from build123d import *

# Parameters (mm, degrees)
P_IDAT_VYSUNUT_M1_DEPTH      = 42
SKICA7_W                     = 10
SKICA7_H                     = 6
P_IDAT_VYSUNUT_M2_DEPTH      = 10
SKICA8_R                     = 3
ODEBRAT_VYSUNUT_M4_DEPTH     = 3
SKICA9_R                     = 1.55
ODEBRAT_VYSUNUT_M5_DEPTH     = 3
LINPOLE1_COUNT               = 2
LINPOLE1_PITCH               = 43
KRUHOV_POLE1_COUNT           = 4
KRUHOV_POLE1_COPY_1_SKETCH_W = 10
KRUHOV_POLE1_COPY_1_SKETCH_H = 6
KRUHOV_POLE1_COPY_1_DEPTH    = 10
KRUHOV_POLE1_COPY_2_SKETCH_W = 10
KRUHOV_POLE1_COPY_2_SKETCH_H = 6
KRUHOV_POLE1_COPY_2_DEPTH    = 10
KRUHOV_POLE1_COPY_3_SKETCH_W = 10
KRUHOV_POLE1_COPY_3_SKETCH_H = 6
KRUHOV_POLE1_COPY_3_DEPTH    = 10
KRUHOV_POLE1_COPY_4_SKETCH_R = 3
KRUHOV_POLE1_COPY_4_DEPTH    = 3
KRUHOV_POLE1_COPY_5_SKETCH_R = 3
KRUHOV_POLE1_COPY_5_DEPTH    = 3
KRUHOV_POLE1_COPY_6_SKETCH_R = 3
KRUHOV_POLE1_COPY_6_DEPTH    = 3
KRUHOV_POLE1_COPY_7_SKETCH_R = 1.55
KRUHOV_POLE1_COPY_7_DEPTH    = 3
KRUHOV_POLE1_COPY_8_SKETCH_R = 1.55
KRUHOV_POLE1_COPY_8_DEPTH    = 3
KRUHOV_POLE1_COPY_9_SKETCH_R = 1.55
KRUHOV_POLE1_COPY_9_DEPTH    = 3
ZAOBLIT3_R                   = 2


with BuildPart() as part:
    # Skica2 → Přidat vysunutím1 (new body)
    with BuildSketch(Plane.XY):
        with BuildLine():
            Line((3, 0), (110, 0))
            ThreePointArc((110, 0), (112.121320344, -0.878679656), (113, -3))
            Line((113, -3), (113, -110))
            ThreePointArc((113, -110), (112.121320344, -112.121320344), (110, -113))
            Line((110, -113), (3, -113))
            ThreePointArc((3, -113), (0.878679656, -112.121320344), (0, -110))
            Line((0, -110), (0, -3))
            ThreePointArc((0, -3), (0.878679656, -0.878679656), (3, 0))
        make_face()
        with BuildLine():
            Line((1, -3), (1, -110))
            ThreePointArc((1, -110), (1.585786438, -111.414213562), (3, -112))
            Line((3, -112), (110, -112))
            ThreePointArc((110, -112), (111.414213562, -111.414213562), (112, -110))
            Line((112, -110), (112, -3))
            ThreePointArc((112, -3), (111.414213562, -1.585786438), (110, -1))
            Line((110, -1), (3, -1))
            ThreePointArc((3, -1), (1.585786438, -1.585786438), (1, -3))
        make_face(mode=Mode.SUBTRACT)
    extrude(amount=P_IDAT_VYSUNUT_M1_DEPTH)

    # Skica7 → Přidat vysunutím2 (add)
    with BuildSketch(Plane(origin=(0, 0, 0), x_dir=(1, 0, 0), z_dir=(0, 1, 0))):
        with Locations((35, -3)):
            Rectangle(SKICA7_W, SKICA7_H)
    p_idat_vysunut_m2 = extrude(amount=P_IDAT_VYSUNUT_M2_DEPTH)

    # Skica8 → Odebrat vysunutím4 (cut)
    with BuildSketch(Plane.XY.offset(6)):
        with Locations((35, 5)):
            Circle(SKICA8_R)
    odebrat_vysunut_m4 = extrude(amount=-ODEBRAT_VYSUNUT_M4_DEPTH, mode=Mode.SUBTRACT)

    # Skica9 → Odebrat vysunutím5 (cut)
    with BuildSketch(Plane.XY.offset(3)):
        with Locations((35, 5)):
            Circle(SKICA9_R)
    odebrat_vysunut_m5 = extrude(amount=-ODEBRAT_VYSUNUT_M5_DEPTH, mode=Mode.SUBTRACT)

    # LinPole1: Přidat vysunutím2, Odebrat vysunutím4, Odebrat vysunutím5 ×2
    with Locations(*[(i * LINPOLE1_PITCH, 0, 0) for i in range(1, LINPOLE1_COUNT)]):
        add(p_idat_vysunut_m2)
        add(odebrat_vysunut_m4, mode=Mode.SUBTRACT)
        add(odebrat_vysunut_m5, mode=Mode.SUBTRACT)

    # Kruhové pole1: Přidat vysunutím2, Odebrat vysunutím4, Odebrat vysunutím5 ×4 about axis
    kruhov_pole1_axis = Axis((56.5, -56.5, 0), (0, 0, 1))
    for i in range(1, KRUHOV_POLE1_COUNT):
        add(p_idat_vysunut_m2.rotate(kruhov_pole1_axis, i * 360 / KRUHOV_POLE1_COUNT))
        add(odebrat_vysunut_m4.rotate(kruhov_pole1_axis, i * 360 / KRUHOV_POLE1_COUNT), mode=Mode.SUBTRACT)
        add(odebrat_vysunut_m5.rotate(kruhov_pole1_axis, i * 360 / KRUHOV_POLE1_COUNT), mode=Mode.SUBTRACT)

    # Kruhové pole1 copy 1 sketch → Kruhové pole1 copy 1 (add)
    with BuildSketch(Plane(origin=(0, -70, 0), x_dir=(0, 1, 0), z_dir=(-1, 0, 0))):
        with Locations((35, -3)):
            Rectangle(KRUHOV_POLE1_COPY_1_SKETCH_W, KRUHOV_POLE1_COPY_1_SKETCH_H)
    extrude(amount=KRUHOV_POLE1_COPY_1_DEPTH)

    # Kruhové pole1 copy 2 sketch → Kruhové pole1 copy 2 (add)
    with BuildSketch(Plane(origin=(70, -113, 0), x_dir=(-1, 0, 0), z_dir=(0, -1, 0))):
        with Locations((35, -3)):
            Rectangle(KRUHOV_POLE1_COPY_2_SKETCH_W, KRUHOV_POLE1_COPY_2_SKETCH_H)
    extrude(amount=KRUHOV_POLE1_COPY_2_DEPTH)

    # Kruhové pole1 copy 3 sketch → Kruhové pole1 copy 3 (add)
    with BuildSketch(Plane(origin=(113, -43, 0), x_dir=(0, -1, 0), z_dir=(1, 0, 0))):
        with Locations((35, -3)):
            Rectangle(KRUHOV_POLE1_COPY_3_SKETCH_W, KRUHOV_POLE1_COPY_3_SKETCH_H)
    extrude(amount=KRUHOV_POLE1_COPY_3_DEPTH)

    # Kruhové pole1 copy 4 sketch → Kruhové pole1 copy 4 (cut)
    with BuildSketch(Plane(origin=(0, -70, 6), x_dir=(0, 1, 0), z_dir=(0, 0, 1))):
        with Locations((35, 5)):
            Circle(KRUHOV_POLE1_COPY_4_SKETCH_R)
    extrude(amount=-KRUHOV_POLE1_COPY_4_DEPTH, mode=Mode.SUBTRACT)

    # Kruhové pole1 copy 5 sketch → Kruhové pole1 copy 5 (cut)
    with BuildSketch(Plane(origin=(70, -113, 6), x_dir=(-1, 0, 0), z_dir=(0, 0, 1))):
        with Locations((35, 5)):
            Circle(KRUHOV_POLE1_COPY_5_SKETCH_R)
    extrude(amount=-KRUHOV_POLE1_COPY_5_DEPTH, mode=Mode.SUBTRACT)

    # Kruhové pole1 copy 6 sketch → Kruhové pole1 copy 6 (cut)
    with BuildSketch(Plane(origin=(113, -43, 6), x_dir=(0, -1, 0), z_dir=(0, 0, 1))):
        with Locations((35, 5)):
            Circle(KRUHOV_POLE1_COPY_6_SKETCH_R)
    extrude(amount=-KRUHOV_POLE1_COPY_6_DEPTH, mode=Mode.SUBTRACT)

    # Kruhové pole1 copy 7 sketch → Kruhové pole1 copy 7 (cut)
    with BuildSketch(Plane(origin=(0, -70, 3), x_dir=(0, 1, 0), z_dir=(0, 0, 1))):
        with Locations((35, 5)):
            Circle(KRUHOV_POLE1_COPY_7_SKETCH_R)
    extrude(amount=-KRUHOV_POLE1_COPY_7_DEPTH, mode=Mode.SUBTRACT)

    # Kruhové pole1 copy 8 sketch → Kruhové pole1 copy 8 (cut)
    with BuildSketch(Plane(origin=(70, -113, 3), x_dir=(-1, 0, 0), z_dir=(0, 0, 1))):
        with Locations((35, 5)):
            Circle(KRUHOV_POLE1_COPY_8_SKETCH_R)
    extrude(amount=-KRUHOV_POLE1_COPY_8_DEPTH, mode=Mode.SUBTRACT)

    # Kruhové pole1 copy 9 sketch → Kruhové pole1 copy 9 (cut)
    with BuildSketch(Plane(origin=(113, -43, 3), x_dir=(0, -1, 0), z_dir=(0, 0, 1))):
        with Locations((35, 5)):
            Circle(KRUHOV_POLE1_COPY_9_SKETCH_R)
    extrude(amount=-KRUHOV_POLE1_COPY_9_DEPTH, mode=Mode.SUBTRACT)

    # Zaoblit3
    zaoblit3_edges = [part.edges().sort_by_distance(p)[0] for p in [
        (83, -113, 3),
        (73, -113, 3),
        (83, -123, 3),
        (73, -123, 3),
        (0, -83, 3),
        (0, -73, 3),
        (-10, -83, 3),
        (-10, -73, 3),
        (113, -73, 3),
        (113, -83, 3),
        (123, -73, 3),
        (123, -83, 3),
        (40, -113, 3),
        (30, -113, 3),
        (40, -123, 3),
        (30, -123, 3),
        (0, -40, 3),
        (0, -30, 3),
        (-10, -40, 3),
        (-10, -30, 3),
        (30, 0, 3),
        (40, 0, 3),
        (30, 10, 3),
        (40, 10, 3),
        (73, 0, 3),
        (83, 0, 3),
        (73, 10, 3),
        (83, 10, 3),
        (113, -30, 3),
        (113, -40, 3),
        (123, -30, 3),
        (123, -40, 3),
    ]]
    fillet(zaoblit3_edges, radius=ZAOBLIT3_R)


solid = part.part
Verification items for the finished model (mm, model axes). A direction names the side the tool comes from. Coordinates: 2 decimals unless noted, no trailing zeros. Order: outer loops, then holes, each group sorted by start corner. A loop starts at its lowest first (then second) coordinate and runs counter-clockwise, first axis right, second up.
1. Scan lines: line 1 (X direction, y = -78, z = 4.1); line 2 (Y direction, x = -5, z = 1.7); line 3 (X direction, y = -35, z = 0.9). Record each from-to range of solid material in increasing order.
Results found:
line 1: x = -10 to -8, -2 to 1, 112 to 115, 121 to 123
line 2: y = -83 to -79.55, -76.45 to -73, -40 to -36.55, -33.45 to -30
line 3: x = -10 to -6.55, -3.45 to 1, 112 to 116.45, 119.55 to 123
2. Sectioned sample at A-A, the plane x = 6.5. Record the cut outline in (y, z), and give its area (3 significant figures).
Results found:
outline: (-113, 0) - (-112, 0) - (-112, 42) - (-113, 42) - close; (-1, 0) - (0, 0) - (0, 42) - (-1, 42) - close
area: 84.0 mm2
3. Sectioned sample at C-C, the plane x = 78. Record the cut outline in (y, z), and give its area (3 significant figures).
Results found:
outline: (-123, 0) - (-119.55, 0) - (-119.55, 3) - (-121, 3) - (-121, 6) - (-123, 6) - close; (-116.45, 0) - (-112, 0) - (-112, 42) - (-113, 42) - (-113, 6) - (-115, 6) - (-115, 3) - (-116.45, 3) - close; (-1, 0) - (3.45, 0) - (3.45, 3) - (2, 3) - (2, 6) - (0, 6) - (0, 42) - (-1, 42) - close; (6.55, 0) - (10, 0) - (10, 6) - (8, 6) - (8, 3) - (6.55, 3) - close
area: 149 mm2
4. Sectioned sample at D-D, the plane z = 37. Record the cut outline in (x, y), and give its area (3 significant figures).
Results found:
outline: (0, -110) arc R3 ccw to (3, -113) - (110, -113) arc R3 ccw to (113, -110) - (113, -3) arc R3 ccw to (110, 0) - (3, 0) arc R3 ccw to (0, -3) - close; hole (1, -110) arc R2 ccw to (3, -112) - (110, -112) arc R2 ccw to (112, -110) - (112, -3) arc R2 ccw to (110, -1) - (3, -1) arc R2 ccw to (1, -3) - close
area: 444 mm2
5. Sectioned sample at B-B, the plane y = -78. Record the cut outline in (x, z), and give its area (3 significant figures).
Results found:
outline: (-10, 0) - (-6.55, 0) - (-6.55, 3) - (-8, 3) - (-8, 6) - (-10, 6) - close; (-3.45, 0) - (1, 0) - (1, 42) - (0, 42) - (0, 6) - (-2, 6) - (-2, 3) - (-3.45, 3) - close; (112, 0) - (116.45, 0) - (116.45, 3) - (115, 3) - (115, 6) - (113, 6) - (113, 42) - (112, 42) - close; (119.55, 0) - (123, 0) - (123, 6) - (121, 6) - (121, 3) - (119.55, 3) - close
area: 149 mm2
6. Go/stop test with flat-tipped pins: pin 1 Ø12 at (x, z) = (62.5, 27.5) entering from +Y; pin 2 Ø12.5 at (y, z) = (-82, 21.5) entering from -X; pin 3 Ø1.5 at (x, z) = (20.5, 19.5) entering from -Y. Record where each tip stops, or that it passes through.
Results found:
pin 1: stops at y = 0
pin 2: stops at x = 0
pin 3: stops at y = -113
7. Release check for a two-part mould opening along Y. For faces 1 (the face through (-5, -83, 3)), 2 (the face through (-3.7, -76.7, 3)), 3 (the face through (-3.2, -80.4, 4.5)), 4 (the face through (118, -30, 3)) record: +Y half, -Y half, draft (parallel to the pull), parting line (faces both ways), or undercut.
Results found:
face 1: -Y half
face 2: undercut
face 3: undercut
face 4: +Y half
8. Set-up check for faces 5 (the face through (81.2, -117.9, 6)), 6 (the face through (32, 5, 5)), 7 (the face through (30, -118, 3)), 8 (the face through (-5, -40, 3)), 9 (the face through (117.9, -31.8, 6)): record each of +Z, -Z, +X, -X, +Y, -Y from which the full face is reachable in a straight line by a thin tool's end or side.
Results found:
face 5: +Z, +X, -X, -Y
face 6: +Z
face 7: +Z, -Z, -X, -Y
face 8: +Z, -Z, -X
face 9: +Z, +X, +Y, -Y
